```python
from build123d import *

# Parameters (mm, degrees)
SKETCH1_R           = 15
BOSS_EXTRUDE1_DEPTH = 63
SKETCH3_R           = 4
BOSS_EXTRUDE2_DEPTH = 10


with BuildPart() as part:
    # Sketch1 → Boss-Extrude1 (new body)
    with BuildSketch(Plane(origin=(0, 0, 0), x_dir=(1, 0, 0), z_dir=(0, 1, 0))):
        Circle(SKETCH1_R)
    extrude(amount=BOSS_EXTRUDE1_DEPTH)

    # Sketch3 → Boss-Extrude2 (add, symmetric)
    with BuildSketch(Plane.XY):
        with BuildLine():
            Line((-13, 0), (-13, -15))
            ThreePointArc((-13, -15), (0, -28), (13, -15))
            Line((13, -15), (13, 0))
            Line((13, 0), (-13, 0))
        make_face()
        with Locations((0, -17)):
            Circle(SKETCH3_R, mode=Mode.SUBTRACT)
        with BuildLine():
            Line((-15, 63), (15, 63))
            Line((15, 63), (15, 69.922962794))
            ThreePointArc((15, 69.922962794), (11.539392014, 78.75472366), (3, 82.88444419))
            ThreePointArc((3, 82.88444419), (0, 83), (-3, 82.88444419))
            ThreePointArc((-3, 82.88444419), (-11.539392014, 78.75472366), (-15, 69.922962794))
            Line((-15, 69.922962794), (-15, 63))
        make_face()
        with Locations((0, 75)):
            Circle(SKETCH3_R, mode=Mode.SUBTRACT)
    extrude(amount=BOSS_EXTRUDE2_DEPTH, both=True)


solid = part.part
```
CAD build for the part. Positions are in the model's coordinates, mm. A direction names the side the tool comes from. Round coordinates to 2 decimals unless told otherwise and drop trailing zeros. Loops run counter-clockwise (first coordinate to the right, second up) from the corner with the lowest first, then second, coordinate; pieces in that order, holes last. Notation, with made-up numbers: (19, 80.25) - (55, 80.25) arc R11 cw to (55, 99.25) - close; hole circle Ø5 at (-10, -39.75). An arc over 180 degrees is marked (long way). Return JSON: item names as keys, results as strings. Group by question number.
Q1. Band-saw the part on D-D on y = 23.5. Give the cut face in (x, z).
Q2. Flat gauge pins, fed straight in: pin 1 Ø4 at (y, z) = (39.5, -7.5) entering from -X; pin 2 Ø3 at (x, z) = (-13, -6.5) entering from -Y; pin 3 Ø5 at (y, z) = (25.5, -7.5) entering from +X. Where does each tip first touch, or does it go through?
Q3. Tool access for faces 5 (the face through (0, 63, -12)), 6 (the face through (0, -11, -10)), 7 (the face through (-13, -7, 0)): list every direction of +Z, -Z, +X, -X, +Y, -Y with a clear straight run to the whole face (end or side of a thin tool).
Q4. Band-saw the part on C-C on x = -7. Give the cut face in (y, z).
Q5. Drill centre lines: line 1 along Y through (x, z) = (0, 2.5); line 2 along Y through (x, z) = (-2, -8.25); line 3 along Z through (x, y) = (10, -6.5). Where is each one in solid material? Low to high. Write a range as [from, to].
Q6. Band-saw the part on B-B on z = 2. Give the cut face in (x, y), plus the area to 3 significant figures.
Q7. Band-saw the part on A-A on y = -17. Give the cut face in (x, z), plus the area to 3 significant figures.
Q8. Two-plate mould, pull along Y, no slides. Class faces 1 (the face through (15, 66, 0)), 2 (the face through (0, 83, 0)), 3 (the face through (-14, 63, 8)), 4 (the face through (0, -28, 0)): +Y half, -Y half, draft (parallel to the pull), parting line (faces both ways), or undercut.
Solutions:
{
 "1": {"outline": "circle Ø30 at (0, 0)"},
 "2": {"pin 1": "stops at x = -13.96", "pin 2": "stops at y = -21.06", "pin 3": "stops at x = 14.14"},
 "3": {"face 5": "-Z, +X, -X, +Y", "face 6": "-Z, +X, -X, -Y", "face 7": "+Z, -Z, -X, -Y"},
 "4": {"outline": "(-25.95, -10) - (0, -10) - (0, -13.27) - (63, -13.27) - (63, -10) - (81.92, -10) - (81.92, 10) - (63, 10) - (63, 13.27) - (0, 13.27) - (0, 10) - (-25.95, 10) - close"},
 "5": {"line 1": "y = [-28, -21], [-13, 71], [79, 83]", "line 2": "y = [-27.85, -20.46], [-13.54, 71.54], [78.46, 82.95]", "line 3": "z = [-10, 10]"},
 "6": {"outline": "(-15, 63) - (-14.87, 63) - (-14.87, 0) - (-13, 0) - (-13, -15) arc R13 ccw to (13, -15) - (13, 0) - (14.87, 0) - (14.87, 63) - (15, 63) - (15, 69.92) arc R13 ccw to (3, 82.88) arc R39 ccw to (-3, 82.88) arc R13 ccw to (-15, 69.92) - close; hole circle Ø8 at (0, -17); hole circle Ø8 at (0, 75)", "area": "2,950 mm^2"},
 "7": {"outline": "(-12.85, -10) - (-4, -10) - (-4, 10) - (-12.85, 10) - close; (4, -10) - (12.85, -10) - (12.85, 10) - (4, 10) - close", "area": "354 mm^2"},
 "8": {"face 1": "draft", "face 2": "+Y half", "face 3": "undercut", "face 4": "-Y half"}
}
